Part print with two shaded views. Sizes in mm from the minimum x, y, z corner. A direction names the side the tool comes from. Give positions to 0.01 mm unless a question says otherwise; leave off trailing zeros. Write each loop counter-clockwise with the first axis right and the second up, starting at its lowest first coordinate (ties: lowest second). Pieces come first, ordered by that corner, then holes.
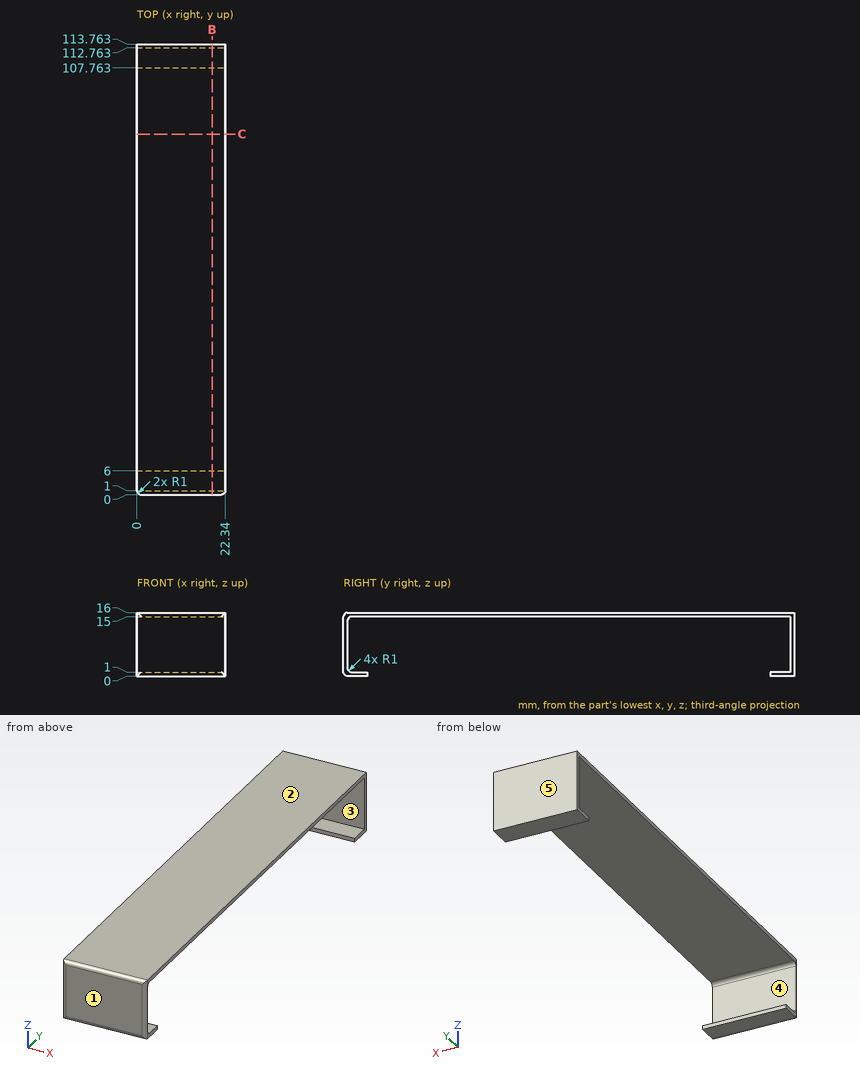
1) Pin check, flat tips, straight feed: pin 1 Ø0.8 at (x, z) = (6, 0.5) entering from -Y (3 decimals); pin 2 Ø4 at (y, z) = (71.5, 11.5) entering from -X. Stop position of each tip, or through.
Answers follow:
pin 1: stops at y = 0.005
pin 2: passes through
2) Wall check: L1, parallel to Y at x = 17.5, z = 2; L2, parallel to Z at x = 3, y = 17; L3, parallel to Y at x = 21.75, z = 2.25. Give the ranges that are in metal, low to high.
Answers follow:
L1: y = 0 to 1, 112.76 to 113.76
L2: z = 15 to 16
L3: y = 0.09 to 1, 112.76 to 113.76
3) 3-axis set-ups, long thin cutter, end or side, ignore diameter. For the marked faces 4 and 5: which of +Z, -Z, +X, -X, +Y, -Y reach the whole face in a straight line?
Answers follow:
face 4: +X, -X
face 5: +Z, -Z, +X, -X, +Y
4) Saw through at C-C, the plane y = 91. Write the cut outline in (x, z).
Answers follow:
outline: (0, 15) - (22.34, 15) - (22.34, 16) - (0, 16) - close
5) Saw through at B-B, the plane x = 19. Write the cut outline in (y, z).
Answers follow:
outline: (0, 1) arc R1 ccw to (1, 0) - (6, 0) - (6, 1) - (2, 1) arc R1 cw to (1, 2) - (1, 14) arc R1 cw to (2, 15) - (112.76, 15) - (112.76, 1) - (107.76, 1) - (107.76, 0) - (113.76, 0) - (113.76, 16) - (1, 16) arc R1 ccw to (0, 15) - close
6) Two-plate mould, pull along Y, no slides. Class the marked faces 1, 2 and 3: +Y half, -Y half, draft (parallel to the pull), parting line (faces both ways), or undercut.
Answers follow:
face 1: -Y half
face 2: draft
face 3: undercut
